```python
from build123d import *

# Parameters (mm, degrees)
F0_W     = 36.510132
F0_H     = 44.657022
F1_DEPTH = 76.2
F2_W     = 44.885072
F2_H     = 44.793312
F3_DEPTH = 103.585832


with BuildPart() as f1:
    # F0 (on Front) → F1 (new body)
    with BuildSketch(Plane.XZ):
        with Locations((-18.255066, -22.328511)):
            Rectangle(F0_W, F0_H)
    extrude(amount=-F1_DEPTH)

    # F2 (on Right) → F3 (join)
    with BuildSketch(Plane.YZ):
        with Locations((-22.442536, -22.396656)):
            Rectangle(F2_W, F2_H)
    extrude(amount=-F3_DEPTH)


solid = f1.part
```
Can you work these out from the model? Positions are in its coordinate system, mm. A direction names the side the tool comes from. Coordinates: 2 decimals unless noted, no trailing zeros. Loops run counter-clockwise (first coordinate to the right, second up) from the corner with the lowest first, then second, coordinate; pieces in that order, holes last.
Item 1: Please list where these lines run through material, in increasing order: L1, parallel to X at y = 9, z = -17.5; L2, parallel to Z at x = -22, y = 67; L3, parallel to Y at x = -67, z = -32.
Answers below:
L1: x = -36.51 to 0
L2: z = -44.66 to 0
L3: y = -44.89 to 0
Item 2: Suppose I cut it at B-B (y = 48). Please give me the cut outline in (x, z), then the cut area to 3 significant figures.
Answers below:
outline: (-36.51, -44.66) - (0, -44.66) - (0, 0) - (-36.51, 0) - close
area: 1,630 mm2
Item 3: Suppose I cut it at A-A (z = -19.5). Please give me the cut outline in (x, y).
Answers below:
outline: (-103.59, -44.89) - (0, -44.89) - (0, 76.2) - (-36.51, 76.2) - (-36.51, 0) - (-103.59, 0) - close
Item 4: Suppose I cut it at C-C (x = -64.5). Please give me the cut outline in (y, z).
Answers below:
outline: (-44.89, -44.79) - (0, -44.79) - (0, 0) - (-44.89, 0) - close
Item 5: I'm going to push flat-ended pins straight in: pin 1 (13.5 mm diameter, centred on y = 41, z = -22.5, fed in from -X); pin 2 (11 mm diameter, centred on x = -16, y = 28.5, fed in from -Z); pin 3 (8 mm diameter, centred on x = -63, z = -23.5, fed in from +Y). Where does each tip first touch, or does it pass through?
Answers below:
pin 1: stops at x = -36.51
pin 2: stops at z = -44.66
pin 3: stops at y = 0
Item 6: Which directions (+Z, -Z, +X, -X, +Y, -Y) give clear straight access to the entire face, cutting with the end or side of a thin tool? Please do faces 1 (the face through (-19, 38, -44.657)), 2 (the face through (-51, -44.885, -23)), 3 (the face through (-36.51, 38, -23)).
Answers below:
face 1: -Z, +X, -X, +Y
face 2: +Z, -Z, +X, -X, -Y
face 3: +Z, -Z, -X, +Y
